Build history of the part. All positions in model axes, mm. Face numbers are marked on the shaded views. A direction names the side the tool comes from. Give positions to 0.01 mm unless a question says otherwise; leave off trailing zeros. Order: outer loops, then holes, each group sorted by start corner. A loop starts at its lowest first (then second) coordinate and runs counter-clockwise, first axis right, second up. Notation, with made-up numbers: M 38.25,58.25 L 71.25,58.25 A22 cw 71.25,78.25 Z; hole C -12.5,6.5 d4. An arc over 180 degrees is marked long. One line per item, written item: value. Start each with the question number.
from build123d import *

# Parameters (mm, degrees)
M2X0_4_TAPPED_HOLE1_D = 1.6
CIRPATTERN1_COUNT     = 6
SKETCH7_W             = 0.5
SKETCH7_H             = 1


with BuildPart() as part:
    # Sketch3 → Main Base (revolve)
    with BuildSketch(Plane(origin=(0, 0, 0), x_dir=(0, 0, -1), z_dir=(1, 0, 0)), mode=Mode.PRIVATE) as main_base_sk:
        with BuildLine():
            Line((0, 24.479181), (33.202143, 24.47918))
            ThreePointArc((33.202143, 24.47918), (49.748007926, 22.300875558), (65.1662995, 15.914410079))
            Line((65.1662995, 15.914410079), (80.000916, 7.349641))
            ThreePointArc((80.000916, 7.349641), (82.214883341, 6.432585552), (84.590763, 6.119795))
            ThreePointArc((84.590763, 6.119795), (84.954745401, 6.148304311), (85.309850177, 6.233136896))
            add(Edge.make_bspline(
                [(85.309850177, 6.233136896), (101.510458516, 11.470300103), (105.161240485, 12.486702482)],
                knots=[0, 0, 0, 1, 1, 1], degree=2))
            Line((105.161240485, 12.486702482), (105.161240485, 17.5))
            Line((105.161240485, 17.5), (103.161240485, 17.5))
            Line((103.161240485, 17.5), (103.161240485, 12.905109467))
            Line((103.161240485, 12.905109467), (84.9926914, 7.181670879))
            ThreePointArc((84.9926914, 7.181670879), (84.794089673, 7.135403418), (84.590762984, 7.119860535))
            ThreePointArc((84.590762984, 7.119860535), (82.473734699, 7.398570567), (80.500976308, 8.215707259))
            Line((80.500976308, 8.215707259), (65.666086023, 16.780559888))
            ThreePointArc((65.666086023, 16.780559888), (50.0067079, 23.266834324), (33.202143, 25.479181))
            Line((33.202143, 25.479181), (2, 25.479181))
            Line((2, 25.479181), (2, 33))
            Line((2, 33), (-4, 33))
            Line((-4, 33), (-4, 32))
            Line((-4, 32), (0, 32))
            Line((0, 32), (0, 24.479181))
        make_face()
    revolve(main_base_sk.sketch.rotate(Axis((0, 0, 0), (0, 0, -1)), 90), axis=Axis((0, 0, 0), (0, 0, -1)))

    # M2x0.4 Tapped Hole1 (through all)
    with Locations(Plane.XY):
        with Locations((0, 29)):
            m2x0_4_tapped_hole1 = Hole(M2X0_4_TAPPED_HOLE1_D / 2)

    # CirPattern1: M2x0.4 Tapped Hole1 ×6 about axis
    cirpattern1_axis = Axis((0, 0, 0), (0, 0, 1))
    for i in range(1, CIRPATTERN1_COUNT):
        add(m2x0_4_tapped_hole1.rotate(cirpattern1_axis, i * 360 / CIRPATTERN1_COUNT), mode=Mode.SUBTRACT)

    # Sketch7 → Face O-Ring (revolve, cut)
    with BuildSketch(Plane(origin=(0, 0, 0), x_dir=(0, 0, -1), z_dir=(1, 0, 0)), mode=Mode.PRIVATE) as face_o_ring_sk:
        with Locations((0.25, 26.4791805)):
            Rectangle(SKETCH7_W, SKETCH7_H)
    revolve(face_o_ring_sk.sketch.rotate(Axis((0, 0, 2.686094), (0, 0, -1)), 90), axis=Axis((0, 0, 2.686094), (0, 0, -1)), mode=Mode.SUBTRACT)


solid = part.part
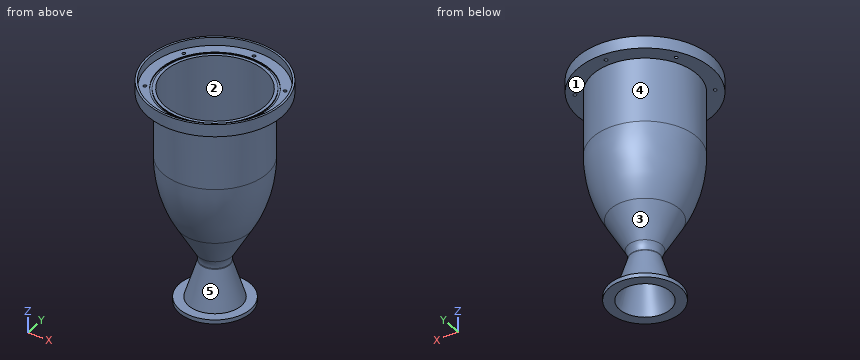
1) Slice it at A-A (z = -21). List the corners of the cut face in (x, y).
2) Drill centre lines: line 1 (X direction, y = 2.5, z = -89.5); line 2 (Z direction, x = -2.5, y = 28.5); line 3 (Y direction, x = 0, z = 2.1). Where is each one in solid material? Low to high.
3) Drop flat-ended pins along their axis: P1, Ø5, axis at y = 11, z = -67, coming from the -X side; P2, Ø6, axis at x = 7.5, z = -8.5, coming from the -Y side; P3, Ø2, axis at x = 0, y = -29, coming from the +Z side; P4, Ø20, axis at x = -10.5, y = 2, coming from the -Z side. Give the stop position or say it passes through.
4) Tool access for the marked faces 4 and 5: list every direction of +Z, -Z, +X, -X, +Y, -Y with a clear straight run to the whole face (end or side of a thin tool).
5) Pull direction Z, two halves, no side cores. Call the marked faces 1, 2 and 3: pulls with the +Z half, pulls with the -Z half, needs draft (parallel to the pull), parting line crosses it, or undercut.
Results list:
1. outline: C 0,0 d50.96; hole C 0,0 d48.96
2. line 1: x = -8.23 to -7.16, 7.16 to 8.23
2. line 2: z = -2 to 0
2. line 3: y = -33 to -32, 32 to 33
3. P1: stops at x = -14.31
3. P2: stops at y = -25.08
3. P3: stops at z = 0
3. P4: stops at z = -105.16
4. face 4: -Z
4. face 5: none
5. face 1: pulls with the -Z half
5. face 2: needs draft
5. face 3: undercut
